from build123d import *

# Parameters (mm, degrees)
DODANIE_WYCI_GNI_CIE1_DEPTH = 5
DODANIE_WYCI_GNI_CIE2_DEPTH = 9
SZKIC4_R                    = 1.45
WYTNIJ_WYCI_GNI_CIE1_DEPTH  = 6


with BuildPart() as part:
    # Szkic1 → Dodanie-wyciągnięcie1 (new body)
    with BuildSketch(Plane(origin=(0, 0, 0), x_dir=(1, 0, 0), z_dir=(0, 1, 0))):
        Polygon((24, 4.5), (27.122498999, 2), (27.122498999, -2), (24, -4.5), (-24, -4.5), (-28, -2), (-28, 2), (-24, 4.5), align=None)
    extrude(amount=DODANIE_WYCI_GNI_CIE1_DEPTH)

    # Szkic2 → Dodanie-wyciągnięcie2 (add)
    with BuildSketch(Plane.XY.offset(4.5)):
        with BuildLine():
            Line((-7.5, 5), (7.5, 5))
            Line((7.5, 5), (7.5, 10.25))
            ThreePointArc((7.5, 10.25), (0, 17.75), (-7.5, 10.25))
            Line((-7.5, 10.25), (-7.5, 5))
        make_face()
    extrude(amount=-DODANIE_WYCI_GNI_CIE2_DEPTH)

    # Szkic4 → Wytnij-wyciągnięcie1 (cut)
    with BuildSketch(Plane(origin=(0, 5, 0), x_dir=(1, 0, 0), z_dir=(0, 1, 0))):
        with Locations(Location((12.40562475, 0, 0), (0, 0, 270))):
            Circle(SZKIC4_R)
        with Locations(Location((21.90562475, 0, 0), (0, 0, 270))):
            Circle(SZKIC4_R)
        with Locations(Location((-12.57201541, 0.053033314, 0), (0, 0, 270))):
            Circle(SZKIC4_R)
        with Locations(Location((-22.71604623, 0.159099943, 0), (0, 0, 270))):
            Circle(SZKIC4_R)
    extrude(amount=-WYTNIJ_WYCI_GNI_CIE1_DEPTH, mode=Mode.SUBTRACT)


solid = part.part
CAD build for the part. Positions are in the model's coordinates, mm. A direction names the side the tool comes from. Give positions to 0.01 mm unless a question says otherwise; leave off trailing zeros. Loops run counter-clockwise (first coordinate to the right, second up) from the corner with the lowest first, then second, coordinate; pieces in that order, holes last. Notation, with made-up numbers: M 76.5,-20.75 L 112.5,-20.75 A18 cw 112.5,-16.75 Z; hole C 40.25,33.25 d9. An arc over 180 degrees is marked long. Answer in a Markdown table with one row per item. Add a question column.
Item 1: Drop flat-ended pins along their axis: P1, Ø4.5, axis at x = 18.5, z = 0, coming from the +Y side; P2, Ø2.5, axis at x = -22.72, z = -0.16, coming from the +Y side; P3, Ø1.6, axis at y = 8.5, z = -2, coming from the +X side; P4, Ø3, axis at y = 13.5, z = -3, coming from the +X side. Give the stop position or say it passes through.
Item 2: Band-saw the part on C-C on y = 9.75. Give the cut face in (x, z), then the cut area to 3 significant figures.
Item 3: Band-saw the part on A-A on z = 0.75. Give the cut face in (x, y), then the cut area to 3 significant figures.
Item 4: Tool access for faces 5 (the face through (17, 5, 0)), 6 (the face through (-7.5, 8, 0)), 7 (the face through (25.5, 2.5, -3.3)): list every direction of +Z, -Z, +X, -X, +Y, -Y with a clear straight run to the whole face (end or side of a thin tool).
Item 5: Band-saw the part on B-B on y = 2.25. Give the cut face in (x, z), then the cut area to 3 significant figures.
Item 6: Mould opens along X. For faces 1 (the face through (13.63, 2.54, 0.78)), 2 (the face through (-28, 2, 0)), 3 (the face through (0, 7, -4.5)), 4 (the face through (-24.132, 2.535, -0.473)) say: +X half, -X half, draft (parallel to the pull), parting line (faces both ways), or undercut.
Item 7: Band-saw the part on D-D on x = 5. Give the cut face in (y, z).
Item 8: Probe probe 1 along X at (y, z) = (3.65, 0); probe 2 along Y at (x, z) = (-9, -3.75); probe 3 along X at (y, z) = (3.5, -0.25). List the from-to ranges inside material, lowest first.
Reply:
| question | item | result |
|---|---|---|
| 1 | P1 | stops at y = 5 |
| 1 | P2 | passes through |
| 1 | P3 | stops at x = 7.5 |
| 1 | P4 | stops at x = 7.29 |
| 2 | outline | M -7.5,-4.5 L 7.5,-4.5 L 7.5,4.5 L -7.5,4.5 Z |
| 2 | area | 135 mm^2 |
| 3 | outline | M -28,0 L -23.85,0 L -23.85,5 L -28,5 Z; M -21.59,0 L -13.78,0 L -13.78,5 L -21.59,5 Z; M -11.36,0 L 11.16,0 L 11.16,5 L 7.5,5 L 7.5,10.25 A7.5 ccw -7.5,10.25 L -7.5,5 L -11.36,5 Z; M 13.65,0 L 20.66,0 L 20.66,5 L 13.65,5 Z; M 23.15,0 L 27.12,0 L 27.12,5 L 23.15,5 Z |
| 3 | area | 395 mm^2 |
| 4 | face 5 | +Z, -Z, +X, +Y |
| 4 | face 6 | +Z, -Z, -X, +Y |
| 4 | face 7 | -Z, +X, +Y, -Y |
| 5 | outline | M -28,-2 L -24,-4.5 L 24,-4.5 L 27.12,-2 L 27.12,2 L 24,4.5 L -24,4.5 L -28,2 Z; hole C -22.72,-0.16 d2.9; hole C -12.57,-0.05 d2.9; hole C 12.41,0 d2.9; hole C 21.91,0 d2.9 |
| 5 | area | 452 mm^2 |
| 6 | face 1 | undercut |
| 6 | face 2 | -X half |
| 6 | face 3 | draft |
| 6 | face 4 | undercut |
| 7 | outline | M 0,-4.5 L 15.84,-4.5 L 15.84,4.5 L 0,4.5 Z |
| 8 | probe 1 | x = -28 to -24.16, -21.27 to -14.02, -11.12 to 10.96, 13.86 to 20.46, 23.36 to 27.12 |
| 8 | probe 2 | y = 0 to 5 |
| 8 | probe 3 | x = -28 to -24.16, -21.27 to -14.01, -11.14 to 10.98, 13.83 to 20.48, 23.33 to 27.12 |
